from build123d import *

# Parameters (mm, degrees)
BOSS_EXTRUDE1_DEPTH     = 10
BOSS_EXTRUDE2_DEPTH     = 2
CUT_EXTRUDE1_REACH      = 23.656
SKETCH5_R               = 1.65
RIB1_REACH              = 26.372
SKETCH4_WALL_W          = 61.924570316
SKETCH4_WALL_H          = 1.5
MIRROR2_COPY_1_REACH    = 26.372
MIRROR2_COPY_1_SKETCH_W = 61.924570316
MIRROR2_COPY_1_SKETCH_H = 1.5


with BuildPart() as part:
    # Sketch2 → Boss-Extrude1 (new body)
    with BuildSketch(Plane.XY):
        with BuildLine():
            Line((1, -0.6), (0, -0.6))
            Line((0, -0.6), (0, -5))
            Line((0, -5), (12, -5))
            Line((12, -5), (12, -15))
            Line((12, -15), (15, -15))
            Line((15, -15), (15, -0.6))
            Line((15, -0.6), (14, -0.6))
            ThreePointArc((14, -0.6), (12.5, -2.1), (11, -0.6))
            Line((11, -0.6), (9, -0.6))
            ThreePointArc((9, -0.6), (7.5, -2.1), (6, -0.6))
            Line((6, -0.6), (4, -0.6))
            ThreePointArc((4, -0.6), (2.5, -2.1), (1, -0.6))
        make_face()
        Polygon((12, 5), (0, 5), (0, 1.3), (15, 1.3), (15, 15), (12, 15), align=None)
        with BuildLine():
            Line((1.215476742, -0.4), (0, -0.4))
            Line((0, -0.4), (0, -0.6))
            Line((0, -0.6), (1, -0.6))
            ThreePointArc((1, -0.6), (2.5, -2.1), (4, -0.6))
            Line((4, -0.6), (6, -0.6))
            ThreePointArc((6, -0.6), (7.5, -2.1), (9, -0.6))
            Line((9, -0.6), (11, -0.6))
            ThreePointArc((11, -0.6), (12.5, -2.1), (14, -0.6))
            Line((14, -0.6), (15, -0.6))
            Line((15, -0.6), (15, -0.4))
            Line((15, -0.4), (13.784523258, -0.4))
            ThreePointArc((13.784523258, -0.4), (12.5, -1.9), (11.215476742, -0.4))
            Line((11.215476742, -0.4), (8.784523258, -0.4))
            ThreePointArc((8.784523258, -0.4), (7.5, -1.9), (6.215476742, -0.4))
            Line((6.215476742, -0.4), (3.784523258, -0.4))
            ThreePointArc((3.784523258, -0.4), (2.5, -1.9), (1.215476742, -0.4))
        make_face()
    extrude(amount=BOSS_EXTRUDE1_DEPTH)

    # Sketch2<4> → Boss-Extrude2 (add)
    with BuildSketch(Plane.XY):
        Polygon((0, 5), (0, -5), (12, -5), (12, -15), (15, -15), (15, 15), (12, 15), (12, 5), align=None)
    extrude(amount=-BOSS_EXTRUDE2_DEPTH)

    # Sketch5 → Cut-Extrude1 (cut, up to next)
    with BuildSketch(Plane.ZY.offset(-12), mode=Mode.PRIVATE) as cut_extrude1_sk1:
        with Locations(Location((4, 10, 0), (0, 0, 270))):
            Circle(SKETCH5_R)
    cut_extrude1_tool1 = extrude(cut_extrude1_sk1.sketch, amount=-CUT_EXTRUDE1_REACH, mode=Mode.PRIVATE) & part.part
    cut_extrude1 = cut_extrude1_tool1.solids().sort_by_distance((12, 10, 4))[0]
    add(cut_extrude1, mode=Mode.SUBTRACT)

    # Sketch4 wall → Rib1 (add, up to next)
    with BuildSketch(Plane(origin=(9.5, 10, 10), x_dir=(0.4472135955, 0.894427191, 0), z_dir=(-0.894427191, 0.4472135955, 0)), mode=Mode.PRIVATE) as rib1_sk1:
        with Locations((0, 0.75)):
            Rectangle(SKETCH4_WALL_W, SKETCH4_WALL_H)
    rib1_tool1 = extrude(rib1_sk1.sketch, amount=-RIB1_REACH, mode=Mode.PRIVATE) - part.part
    rib1 = rib1_tool1.solids().sort_by_distance((9.5, 10, 10))[0]
    add(rib1)

    # Mirror1: Rib1 across plane
    add(rib1.mirror(Plane.XY.offset(4)))

    # Mirror2: Cut-Extrude1, Rib1 across plane
    add(cut_extrude1.mirror(Plane.ZX), mode=Mode.SUBTRACT)
    add(rib1.mirror(Plane.ZX))

    # Mirror2 copy 1 sketch → Mirror2 copy 1 (add, up to next)
    with BuildSketch(Plane(origin=(9.5, -10, -2), x_dir=(0.4472135955, -0.894427191, 0), z_dir=(-0.894427191, -0.4472135955, 0)), mode=Mode.PRIVATE) as mirror2_copy_1_sk1:
        with Locations((0, 0.75)):
            Rectangle(MIRROR2_COPY_1_SKETCH_W, MIRROR2_COPY_1_SKETCH_H)
    mirror2_copy_1_tool1 = extrude(mirror2_copy_1_sk1.sketch, amount=-MIRROR2_COPY_1_REACH, mode=Mode.PRIVATE) - part.part
    add(mirror2_copy_1_tool1.solids().sort_by_distance((9.5, -10, -2))[0])


solid = part.part
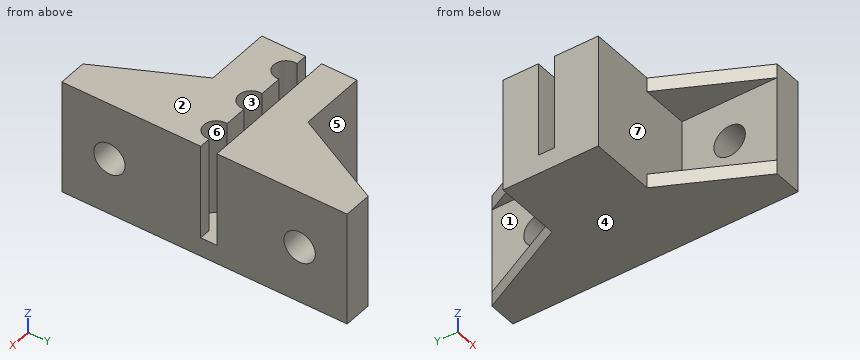
Input: part model. Units: mm. Frame: model coordinates. Face numbers are marked on the shaded views. A direction names the side the tool comes from. Give positions to 0.01 mm unless a question says otherwise; leave off trailing zeros. Write each loop counter-clockwise with the first axis right and the second up, starting at its lowest first coordinate (ties: lowest second). Pieces come first, ordered by that corner, then holes. Notation, with made-up numbers: (-13, 26) -> (15, 26) arc R26 ccw to (15, 44) -> close; hole circle Ø4 at (63.25, 27). An arc over 180 degrees is marked (long way). Use one line per item in the form item = value. Start each with the question number.
1) Set-up query: the marked faces 5, 6 and 7. Return all of +Z, -Z, +X, -X, +Y, -Y with unobstructed straight access to the full face (end or side cutting, diameter ignored); none if empty.
2) Section query A-A on y = 10. Return the cut outline in (x, z).
3) Draft query along Z for the marked faces 1, 2, 3 and 4. Return one class per face: pulls with the +Z half, pulls with the -Z half, needs draft (parallel to the pull), parting line crosses it, or undercut.
4) Pin query (flat end, axial travel): pin 1 (1.5 mm diameter, centred on x = 8.5, y = 10, fed in from +Z); pin 2 (4 mm diameter, centred on y = 10, z = 4, fed in from -X); pin 3 (2.5 mm diameter, centred on x = 10, z = 4, fed in from +Y); pin 4 (1 mm diameter, centred on x = 4.5, z = 5.5, fed in from -Y). Return the tip coordinate at first contact, or that it passes through.
5) Section query D-D on x = 12.5. Return the cut outline in (y, z), then the cut area to 3 significant figures.
6) Ray query, probe 1 along X at (y, z) = (-0.6, 7); probe 2 along Y at (x, z) = (6, 1.25); probe 3 along Y at (x, z) = (8.5, 2.25). Return the intervals inside material, ascending. Write a range as from..to.
7) Section query B-B on z = 0.75. Return the cut outline in (x, y), then the cut area to 3 significant figures.
8) Section query C-C on z = 4. Return the cut outline in (x, y).
Outcome:
q1.face_5 = -X, +Y
q1.face_6 = +Z
q1.face_7 = -X, -Y
q2.outline = (9.5, -2) -> (15, -2) -> (15, 2.35) -> (12, 2.35) -> (12, -0.5) -> (9.5, -0.5) -> close; (9.5, 8.5) -> (12, 8.5) -> (12, 5.65) -> (15, 5.65) -> (15, 10) -> (9.5, 10) -> close
q3.face_1 = undercut
q3.face_2 = pulls with the +Z half
q3.face_3 = needs draft
q3.face_4 = pulls with the -Z half
q4.pin_1 = through
q4.pin_2 = 12
q4.pin_3 = 5
q4.pin_4 = -5
q5.outline = (-15, -2) -> (15, -2) -> (15, 10) -> (1.3, 10) -> (1.3, 0) -> (-1.9, 0) -> (-1.9, 10) -> (-15, 10) -> close; hole circle Ø3.3 at (-10, 4); hole circle Ø3.3 at (10, 4)
q5.area = 311 mm^2
q6.probe_1 = 0..1.2, 3.8..6.2, 8.8..11.2, 13.8..15
q6.probe_2 = -5..-0.4, 1.3..5
q6.probe_3 = -5..-1.43, 1.3..5
q7.outline = (0, -5) -> (12, -5) -> (12, -15) -> (15, -15) -> (15, -0.4) -> (13.78, -0.4) arc R1.3 cw (long way) to (11.22, -0.4) -> (8.78, -0.4) arc R1.3 cw (long way) to (6.22, -0.4) -> (3.78, -0.4) arc R1.3 cw (long way) to (1.22, -0.4) -> (0, -0.4) -> close; (0, 1.3) -> (15, 1.3) -> (15, 15) -> (12, 15) -> (12, 5) -> (0, 5) -> close
q7.area = 175 mm^2
q8.outline = (0, -5) -> (12, -5) -> (12, -8.35) -> (15, -8.35) -> (15, -0.4) -> (13.78, -0.4) arc R1.3 cw (long way) to (11.22, -0.4) -> (8.78, -0.4) arc R1.3 cw (long way) to (6.22, -0.4) -> (3.78, -0.4) arc R1.3 cw (long way) to (1.22, -0.4) -> (0, -0.4) -> close; (0, 1.3) -> (15, 1.3) -> (15, 8.35) -> (12, 8.35) -> (12, 5) -> (0, 5) -> close; (12, -15) -> (15, -15) -> (15, -11.65) -> (12, -11.65) -> close; (12, 11.65) -> (15, 11.65) -> (15, 15) -> (12, 15) -> close
